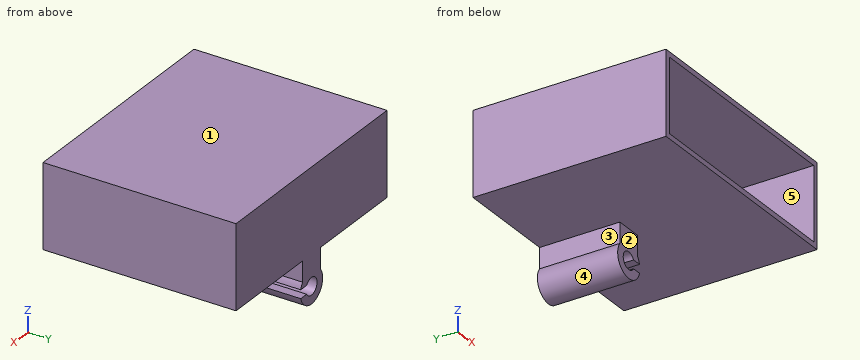
```python
from build123d import *

# Parameters (mm, degrees)
SKETCH_1_W          = 68
SKETCH_1_H          = 56.5
EXTRUDE_1_DEPTH     = 24.5
SKETCH_4_W          = 65.1
SKETCH_4_H          = 21.5
CUT_EXTRUDE_2_DEPTH = 55
SKETCH_6_W          = 8
SKETCH_6_H          = 56.5
EXTRUDE_3_DEPTH     = 6
EXTRUDE_4_DEPTH     = 56.5
SKETCH_9_W          = 19
SKETCH_9_H          = 33
CUT_EXTRUDE_3_DEPTH = 15


with BuildPart() as part:
    # 草图1 → 凸台-拉伸1 (new body)
    with BuildSketch(Plane.XY):
        with Locations((34, -28.25)):
            Rectangle(SKETCH_1_W, SKETCH_1_H)
    extrude(amount=EXTRUDE_1_DEPTH)

    # 草图4 → 切除-拉伸2 (cut)
    with BuildSketch(Plane.XZ.offset(56.5)):
        with Locations((34, 12.25)):
            Rectangle(SKETCH_4_W, SKETCH_4_H)
    extrude(amount=-CUT_EXTRUDE_2_DEPTH, mode=Mode.SUBTRACT)

    # 草图6 → 凸台-拉伸3 (add)
    with BuildSketch(Plane(origin=(0, 0, 0), x_dir=(-1, 0, 0), z_dir=(0, 0, -1))):
        with Locations((-34, -28.25)):
            Rectangle(SKETCH_6_W, SKETCH_6_H)
    extrude(amount=EXTRUDE_3_DEPTH)

    # 草图8 → 凸台-拉伸4 (add)
    with BuildSketch(Plane(origin=(0, 0, 0), x_dir=(1, 0, 0), z_dir=(0, 1, 0))):
        with BuildLine():
            Line((34, 6), (38, 6))
            ThreePointArc((38, 6), (38.50637974, 6.833772488), (38.841229183, 7.75))
            Line((38.841229183, 7.75), (36.165055224, 7.75))
            ThreePointArc((36.165055224, 7.75), (31.500007176, 9), (36.165055224, 10.25))
            Line((36.165055224, 10.25), (38.841229183, 10.25))
            ThreePointArc((38.841229183, 10.25), (31.833772488, 13.50637974), (30, 6))
            Line((30, 6), (34, 6))
        make_face()
    extrude(amount=-EXTRUDE_4_DEPTH)

    # 草图9 → 切除-拉伸3 (cut)
    with BuildSketch(Plane(origin=(0, 0, 0), x_dir=(-1, 0, 0), z_dir=(0, 0, -1))):
        with Locations((-33.897010853, -40)):
            Rectangle(SKETCH_9_W, SKETCH_9_H)
    extrude(amount=CUT_EXTRUDE_3_DEPTH, mode=Mode.SUBTRACT)


solid = part.part
```
Source: CAD feature listing. Evaluate the final solid. Frame: model axes, mm. Face numbers are marked on the shaded views. A direction names the side the tool comes from. Give positions to 0.01 mm unless a question says otherwise; leave off trailing zeros. Order: outer loops, then holes, each group sorted by start corner. A loop starts at its lowest first (then second) coordinate and runs counter-clockwise, first axis right, second up.
(1) Section query A-A (x = 34). Return the cut outline in (y, z).
(2) Section query B-B (y = -21). Return the cut outline in (x, z).
(3) Section query D-D (x = 55.5). Return the cut outline in (y, z).
(4) Contact query for flat-ended pins moving along their axis: P1, Ø3, axis at x = 37.5, y = -8, coming from the -Z side; P2, Ø5, axis at x = 32.5, z = -6.5, coming from the -Y side; P3, Ø17, axis at x = 30, z = 13.5, coming from the -Y side. Output: stop coordinate, or through.
(5) Section query C-C (z = 14). Return the cut outline in (x, y).
(6) Material intervals for line 1 along Z through (x, y) = (34, -6); line 2 along Z through (x, y) = (46, -8.5); line 3 along X through (y, z) = (-48, 20), sorted ascending.
(7) Access query for the marked faces 4 and 5. Directions: +Z, -Z, +X, -X, +Y, -Y. A direction counts if a zero-diameter tool reaches every point of the face in a straight line with its end or side. Return the directions, or none.
(8) Pull-direction query (Z, two-part tool) for the marked faces 1, 2 and 3; classes: +Z half, -Z half, draft (parallel to the pull), parting line (faces both ways), or undercut.
Outcome:
1. outline: (-56.5, 0) - (-23.5, 0) - (-23.5, -6.5) - (0, -6.5) - (0, 24.5) - (-56.5, 24.5) - (-56.5, 23) - (-1.5, 23) - (-1.5, 1.5) - (-56.5, 1.5) - close; (-23.5, -14) - (0, -14) - (0, -11.5) - (-23.5, -11.5) - close
2. outline: (0, 0) - (30, 0) - (30, -6) arc R5 ccw (long way) to (38.84, -10.25) - (36.17, -10.25) arc R2.5 cw (long way) to (36.17, -7.75) - (38.84, -7.75) arc R5 ccw to (38, -6) - (38, 0) - (68, 0) - (68, 24.5) - (0, 24.5) - close; hole (1.45, 1.5) - (66.55, 1.5) - (66.55, 23) - (1.45, 23) - close
3. outline: (-56.5, 0) - (0, 0) - (0, 24.5) - (-56.5, 24.5) - (-56.5, 23) - (-1.5, 23) - (-1.5, 1.5) - (-56.5, 1.5) - close
4. P1: stops at z = -13.58
4. P2: stops at y = -23.5
4. P3: stops at y = -1.5
5. outline: (0, -56.5) - (1.45, -56.5) - (1.45, -1.5) - (66.55, -1.5) - (66.55, -56.5) - (68, -56.5) - (68, 0) - (0, 0) - close
6. line 1: z = -14 to -11.5, -6.5 to 1.5, 23 to 24.5
6. line 2: z = 0 to 1.5, 23 to 24.5
6. line 3: x = 0 to 1.45, 66.55 to 68
7. face 4: +Y, -Y
7. face 5: -Y
8. face 1: +Z half
8. face 2: draft
8. face 3: undercut
